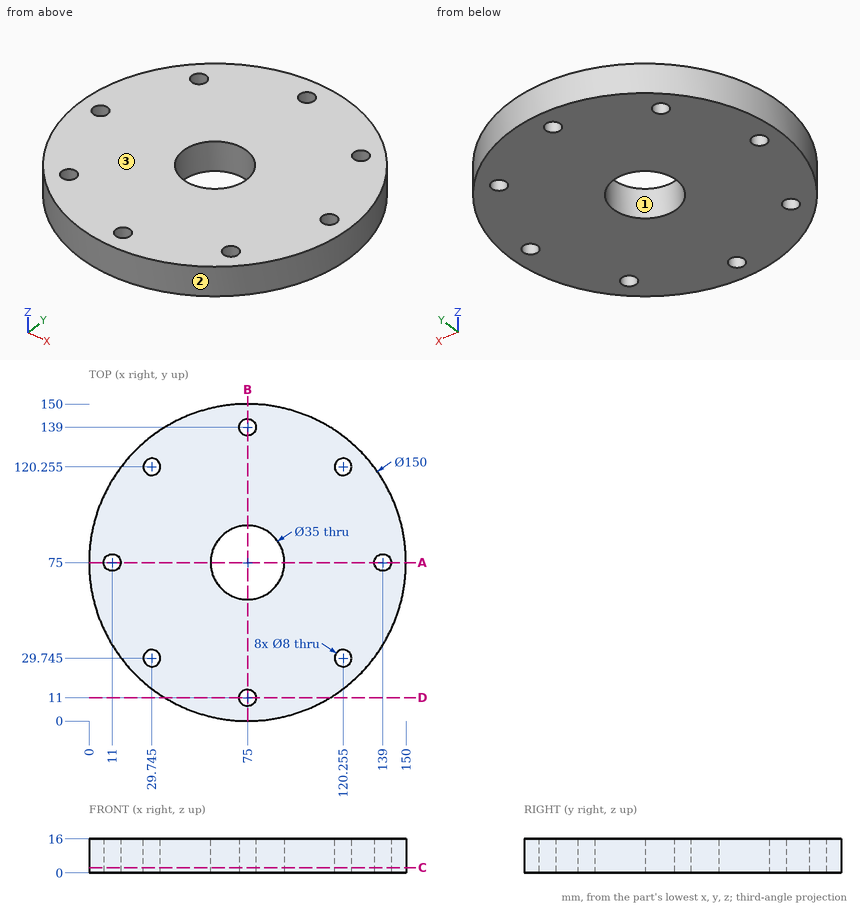
Print and shaded views of the part. All mm, measured from the part's lowest x, y and z. Coordinates: 2 decimals unless noted, no trailing zeros. Order: outer loops, then holes, each group sorted by start corner. A loop starts at its lowest first (then second) coordinate and runs counter-clockwise, first axis right, second up. Notation, with made-up numbers: M 25.25,64 L 66.25,64 A28 ccw 66.25,91 Z; hole C -31,43.25 d11. An arc over 180 degrees is marked long. One line per question, with ' | ' between items. Start each with the question number.
Q1. Two-plate mould, pull along X, no slides. Class the marked faces 1, 2 and 3: +X half, -X half, draft (parallel to the pull), parting line (faces both ways), or undercut.
Q2. Saw through at C-C (z = 2.5). Count the separate pieces of the cut face and the enclosed holes in it, then the cut area to 3 significant figures.
Q3. Saw through at D-D (y = 11). List the corners of the cut face in (x, z), then the cut area to 3 significant figures.
Q4. Flat gauge pins, fed straight in: pin 1 Ø2 at (y, z) = (73, 6) entering from +X; pin 2 Ø3 at (y, z) = (43, 11) entering from +X; pin 3 Ø4 at (y, z) = (20, 10) entering from -X. Where does each tip first touch, or does it go through?
Q5. Saw through at A-A (y = 75). List the corners of the cut face in (x, z).
Q6. Probe L1, parallel to Y at x = 74.5, z = 9; L2, parallel to Y at x = 78, z = 13.5 (1 decimal); L3, parallel to X at y = 86, z = 4. List the from-to ranges inside material, lowest first. Write a range as from..to.
Check values:
1) face 1: undercut | face 2: parting line | face 3: draft
2) separate pieces: 1 | enclosed holes: 9 | area: 16,300 mm2
3) outline: M 35.9,0 L 71,0 L 71,16 L 35.9,16 Z; M 79,0 L 114.1,0 L 114.1,16 L 79,16 Z | area: 1,120 mm2
4) pin 1: stops at x = 149.99 | pin 2: stops at x = 143.52 | pin 3: stops at x = 21.93
5) outline: M 0,0 L 7,0 L 7,16 L 0,16 Z; M 15,0 L 57.5,0 L 57.5,16 L 15,16 Z; M 92.5,0 L 135,0 L 135,16 L 92.5,16 Z; M 143,0 L 150,0 L 150,16 L 143,16 Z
6) L1: y = 0..7.03, 14.97..57.51, 92.49..135.03, 142.97..150 | L2: y = 0.1..8.4, 13.6..57.8, 92.2..136.4, 141.6..149.9 | L3: x = 0.81..61.39, 88.61..149.19
